Build history of the part. All positions in model axes, mm. Face numbers are marked on the shaded views. A direction names the side the tool comes from. Round coordinates to 2 decimals unless told otherwise and drop trailing zeros. Loops run counter-clockwise (first coordinate to the right, second up) from the corner with the lowest first, then second, coordinate; pieces in that order, holes last.
from build123d import *

# Parameters (mm, degrees)
SKETCH1_R           = 25
BOSS_EXTRUDE1_DEPTH = 50
SKETCH2_W           = 10
SKETCH2_H           = 10
BOSS_EXTRUDE2_DEPTH = 10
SKETCH3_R           = 2.5
BOSS_EXTRUDE3_DEPTH = 3
BOSS_EXTRUDE4_START = 3
SKETCH4_R           = 2.5
BOSS_EXTRUDE4_DEPTH = 3
CIRPATTERN1_COUNT   = 3
SKETCH5_R           = 7.5
SKETCH6_R           = 15
FILLET1_R           = 10
FILLET2_R           = 5


with BuildPart() as part:
    # Sketch1 → Boss-Extrude1 (new body)
    with BuildSketch(Plane.XY):
        Circle(SKETCH1_R)
    extrude(amount=BOSS_EXTRUDE1_DEPTH)

    # Sketch2 → Boss-Extrude2 (add)
    with BuildSketch(Plane(origin=(0, 0, 0), x_dir=(-1, 0, 0), z_dir=(0, 0, -1))):
        with Locations((29.494897428, 0)):
            Rectangle(SKETCH2_W, SKETCH2_H)
    boss_extrude2 = extrude(amount=-BOSS_EXTRUDE2_DEPTH)

    # Sketch3 → Boss-Extrude3 (add)
    with BuildSketch(Plane.XZ.offset(5)):
        with Locations((-29.494897428, 5)):
            Circle(SKETCH3_R)
    boss_extrude3 = extrude(amount=BOSS_EXTRUDE3_DEPTH)

    # Sketch4 → Boss-Extrude4 (add)
    with BuildSketch(Plane(origin=(0, 5, 0), x_dir=(1, 0, 0), z_dir=(0, 1, 0)).offset(BOSS_EXTRUDE4_START)):
        with Locations((-29.494897428, -5)):
            Circle(SKETCH4_R)
    boss_extrude4 = extrude(amount=-BOSS_EXTRUDE4_DEPTH)

    # CirPattern1: Boss-Extrude2, Boss-Extrude3, Boss-Extrude4 ×3 about axis
    cirpattern1_axis = Axis((0, 0, 0), (0, 0, 1))
    add([boss_extrude2.rotate(cirpattern1_axis, i * 360 / CIRPATTERN1_COUNT) for i in range(1, CIRPATTERN1_COUNT)])
    add([boss_extrude3.rotate(cirpattern1_axis, i * 360 / CIRPATTERN1_COUNT) for i in range(1, CIRPATTERN1_COUNT)])
    add([boss_extrude4.rotate(cirpattern1_axis, i * 360 / CIRPATTERN1_COUNT) for i in range(1, CIRPATTERN1_COUNT)])

    # Sketch5 → Cut-Loft1 section 0
    with BuildSketch(Plane.XY.offset(50)):
        Circle(SKETCH5_R)
    # Sketch6 → Cut-Loft1 section 1
    with BuildSketch(Plane(origin=(0, 0, 0), x_dir=(-1, 0, 0), z_dir=(0, 0, -1))):
        Circle(SKETCH6_R)
    loft(mode=Mode.SUBTRACT)

    # Fillet1
    fillet1_edges = [part.edges().sort_by_distance(p)[0] for p in [
        (-25, 0, 50),
    ]]
    fillet(fillet1_edges, radius=FILLET1_R)

    # Fillet2
    # the kernel refuses this fillet: 5 mm, written as the material it takes off along each edge
    with BuildSketch(Plane(origin=(0, 0, 0), x_dir=(0.22300738877667003, -0.9748167543446364, 0), z_dir=(-0.9748167543446364, -0.22300738877667003, 0))) as fillet2_piece_1_section:
        with BuildLine():
            CenterArc((25 - FILLET2_R, FILLET2_R), FILLET2_R, 270, 90)
            Line((25 - FILLET2_R, 0), (25, 0))
            Line((25, 0), (25, FILLET2_R))
        make_face()
    fillet2_piece_1 = revolve(axis=Axis((0, 0, 0), (0, 0, 1)), revolution_arc=77.11426693, mode=Mode.PRIVATE)
    fillet2_piece_1 = split(fillet2_piece_1, bisect_by=Plane(origin=(7.29782447, -22.640202767, 1.23109977), z_dir=(-0.8660254037844394, -0.49999999999999883, 0)), keep=Keep.TOP, mode=Mode.PRIVATE)
    add(fillet2_piece_1, mode=Mode.SUBTRACT)
    with BuildSketch(Plane(origin=(0, 0, 0), x_dir=(0.22300738877667003, -0.9748167543446364, 0), z_dir=(-0.9748167543446364, -0.22300738877667003, 0))) as fillet2_piece_2_section:
        with BuildLine():
            CenterArc((25 - FILLET2_R, FILLET2_R), FILLET2_R, 270, 90)
            Line((25 - FILLET2_R, 0), (25, 0))
            Line((25, 0), (25, FILLET2_R))
        make_face()
    fillet2_piece_2 = revolve(axis=Axis((0, 0, 0), (0, 0, 1)), revolution_arc=77.11426693, mode=Mode.PRIVATE)
    fillet2_piece_2 = split(fillet2_piece_2, bisect_by=Plane(origin=(13.725987665, -13.77410802, 1.168109868), z_dir=(0.8660254037844394, 0.4999999999999987, 0)), keep=Keep.TOP, mode=Mode.PRIVATE)
    add(fillet2_piece_2, mode=Mode.SUBTRACT)
    with BuildSketch(Plane(origin=(0, 0, 0), x_dir=(0.732831285228025, 0.68041039629847, 0), z_dir=(0.68041039629847, -0.732831285228025, 0))) as fillet2_piece_3_section:
        with BuildLine():
            CenterArc((25 - FILLET2_R, FILLET2_R), FILLET2_R, 270, 90)
            Line((25 - FILLET2_R, 0), (25, 0))
            Line((25, 0), (25, FILLET2_R))
        make_face()
    fillet2_piece_3 = revolve(axis=Axis((0, 0, 0), (0, 0, 1)), revolution_arc=154.248557626, mode=Mode.PRIVATE)
    fillet2_piece_3 = split(fillet2_piece_3, bisect_by=Plane(origin=(15.957681681, 17.639515442, 1.230959753), z_dir=(0.8660254037844378, -0.5000000000000014, 0)), keep=Keep.TOP, mode=Mode.PRIVATE)
    add(fillet2_piece_3, mode=Mode.SUBTRACT)
    with BuildSketch(Plane(origin=(0, 0, 0), x_dir=(0.732831285228025, 0.68041039629847, 0), z_dir=(0.68041039629847, -0.732831285228025, 0))) as fillet2_piece_4_section:
        with BuildLine():
            CenterArc((25 - FILLET2_R, FILLET2_R), FILLET2_R, 270, 90)
            Line((25 - FILLET2_R, 0), (25, 0))
            Line((25, 0), (25, FILLET2_R))
        make_face()
    fillet2_piece_4 = revolve(axis=Axis((0, 0, 0), (0, 0, 1)), revolution_arc=154.248557626, mode=Mode.PRIVATE)
    fillet2_piece_4 = split(fillet2_piece_4, bisect_by=Plane(origin=(1.564958422, 12.710587499, 1.419658234), z_dir=(-0.8660254037844378, 0.5000000000000017, 0)), keep=Keep.TOP, mode=Mode.PRIVATE)
    fillet2_piece_4 = split(fillet2_piece_4, bisect_by=Plane(origin=(-11.790170883, 5, 1.419658234), z_dir=(0, 1, 0)), keep=Keep.TOP, mode=Mode.PRIVATE)
    add(fillet2_piece_4, mode=Mode.SUBTRACT)
    with BuildSketch(Plane(origin=(0, 0, 0), x_dir=(0.732831285228025, 0.68041039629847, 0), z_dir=(0.68041039629847, -0.732831285228025, 0))) as fillet2_piece_5_section:
        with BuildLine():
            CenterArc((25 - FILLET2_R, FILLET2_R), FILLET2_R, 270, 90)
            Line((25 - FILLET2_R, 0), (25, 0))
            Line((25, 0), (25, FILLET2_R))
        make_face()
    fillet2_piece_5 = revolve(axis=Axis((0, 0, 0), (0, 0, 1)), revolution_arc=154.248557626, mode=Mode.PRIVATE)
    fillet2_piece_5 = split(fillet2_piece_5, bisect_by=Plane(origin=(-23.255109262, -5, 1.230959847), z_dir=(0, -1, 0)), keep=Keep.TOP, mode=Mode.PRIVATE)
    add(fillet2_piece_5, mode=Mode.SUBTRACT)
    with BuildSketch(Plane(origin=(0, 0, 0), x_dir=(-0.9556683308075251, 0.29444531154623416, 0), z_dir=(0.29444531154623416, 0.9556683308075251, 0))) as fillet2_piece_6_section:
        with BuildLine():
            CenterArc((25 - FILLET2_R, FILLET2_R), FILLET2_R, 270, 90)
            Line((25 - FILLET2_R, 0), (25, 0))
            Line((25, 0), (25, FILLET2_R))
        make_face()
    fillet2_piece_6 = revolve(axis=Axis((0, 0, 0), (0, 0, 1)), revolution_arc=154.248557626, mode=Mode.PRIVATE)
    fillet2_piece_6 = split(fillet2_piece_6, bisect_by=Plane(origin=(-23.255109324, 5, 1.230959753), z_dir=(0, 1, 0)), keep=Keep.TOP, mode=Mode.PRIVATE)
    add(fillet2_piece_6, mode=Mode.SUBTRACT)
    with BuildSketch(Plane(origin=(0, 0, 0), x_dir=(-0.9556683308075251, 0.29444531154623416, 0), z_dir=(0.29444531154623416, 0.9556683308075251, 0))) as fillet2_piece_7_section:
        with BuildLine():
            CenterArc((25 - FILLET2_R, FILLET2_R), FILLET2_R, 270, 90)
            Line((25 - FILLET2_R, 0), (25, 0))
            Line((25, 0), (25, FILLET2_R))
        make_face()
    fillet2_piece_7 = revolve(axis=Axis((0, 0, 0), (0, 0, 1)), revolution_arc=154.248557626, mode=Mode.PRIVATE)
    fillet2_piece_7 = split(fillet2_piece_7, bisect_by=Plane(origin=(1.564958422, -12.710587499, 1.419658234), z_dir=(-0.8660254037844394, -0.49999999999999883, 0)), keep=Keep.TOP, mode=Mode.PRIVATE)
    fillet2_piece_7 = split(fillet2_piece_7, bisect_by=Plane(origin=(-11.790170883, -5, 1.419658234), z_dir=(0, -1, 0)), keep=Keep.TOP, mode=Mode.PRIVATE)
    add(fillet2_piece_7, mode=Mode.SUBTRACT)
    with BuildSketch(Plane(origin=(0, 0, 0), x_dir=(-0.9556683308075251, 0.29444531154623416, 0), z_dir=(0.29444531154623416, 0.9556683308075251, 0))) as fillet2_piece_8_section:
        with BuildLine():
            CenterArc((25 - FILLET2_R, FILLET2_R), FILLET2_R, 270, 90)
            Line((25 - FILLET2_R, 0), (25, 0))
            Line((25, 0), (25, FILLET2_R))
        make_face()
    fillet2_piece_8 = revolve(axis=Axis((0, 0, 0), (0, 0, 1)), revolution_arc=154.248557626, mode=Mode.PRIVATE)
    fillet2_piece_8 = split(fillet2_piece_8, bisect_by=Plane(origin=(15.95768165, -17.639515389, 1.230959847), z_dir=(0.8660254037844394, 0.4999999999999987, 0)), keep=Keep.TOP, mode=Mode.PRIVATE)
    add(fillet2_piece_8, mode=Mode.SUBTRACT)
    with BuildSketch(Plane(origin=(0, 0, 0), x_dir=(1, 0, 0), z_dir=(0, -1, 0))) as fillet2_piece_9_section:
        with BuildLine():
            CenterArc((25 - FILLET2_R, FILLET2_R), FILLET2_R, 270, 90)
            Line((25 - FILLET2_R, 0), (25, 0))
            Line((25, 0), (25, FILLET2_R))
        make_face()
    fillet2_piece_9 = revolve(axis=Axis((0, 0, 0), (0, 0, 1)), revolution_arc=77.11426693, mode=Mode.PRIVATE)
    fillet2_piece_9 = split(fillet2_piece_9, bisect_by=Plane(origin=(13.725987546, 13.774107814, 1.168109699), z_dir=(0.8660254037844378, -0.5000000000000014, 0)), keep=Keep.TOP, mode=Mode.PRIVATE)
    add(fillet2_piece_9, mode=Mode.SUBTRACT)
    with BuildSketch(Plane(origin=(0, 0, 0), x_dir=(1, 0, 0), z_dir=(0, -1, 0))) as fillet2_piece_10_section:
        with BuildLine():
            CenterArc((25 - FILLET2_R, FILLET2_R), FILLET2_R, 270, 90)
            Line((25 - FILLET2_R, 0), (25, 0))
            Line((25, 0), (25, FILLET2_R))
        make_face()
    fillet2_piece_10 = revolve(axis=Axis((0, 0, 0), (0, 0, 1)), revolution_arc=77.11426693, mode=Mode.PRIVATE)
    fillet2_piece_10 = split(fillet2_piece_10, bisect_by=Plane(origin=(7.297824439, 22.640202713, 1.231099864), z_dir=(-0.8660254037844378, 0.5000000000000017, 0)), keep=Keep.TOP, mode=Mode.PRIVATE)
    add(fillet2_piece_10, mode=Mode.SUBTRACT)


solid = part.part
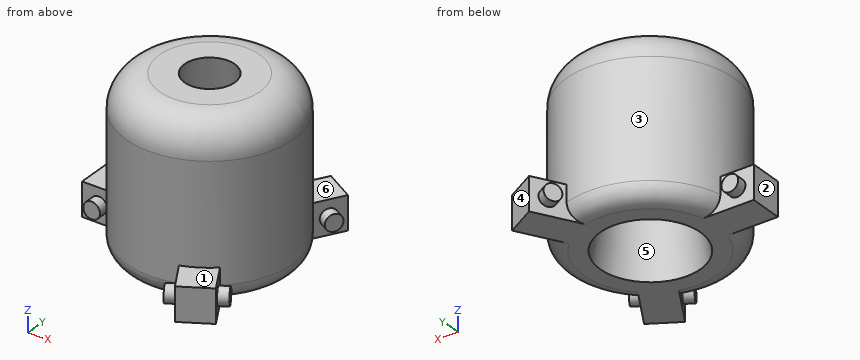
(1) Slice it at C-C on y = 6. Count the separate pieces of the cut face and the enclosed holes in it, plus the area to 3 significant figures.
Responses:
separate pieces: 3
enclosed holes: 0
area: 1,450 mm2
(2) Slice it at D-D on z = 26. List the corners of the cut face in (x, y), plus the area to 3 significant figures.
Responses:
outline: circle Ø50 at (0, 0); hole circle Ø22.2 at (0, 0)
area: 1,580 mm2
(3) Probe line 1 (Z direction, x = 15.5, y = 20.5); line 2 (X direction, y = 8, z = 12.5); line 3 (X direction, y = -6.5, z = 24). List the from-to ranges inside material, lowest first.
Responses:
line 1: z = 0 to 10
line 2: x = -23.69 to -10.41, 10.41 to 23.69
line 3: x = -24.14 to -9.37, 9.37 to 24.14
(4) Slice it at A-A on x = 0. List the corners of the cut face in (y, z).
Responses:
outline: (-25, 5) arc R5 ccw to (-20, 0) - (-15, 0) - (-7.5, 50) - (-15, 50) arc R10 ccw to (-25, 40) - close; (7.5, 50) - (15, 0) - (20, 0) arc R5 ccw to (25, 5) - (25, 40) arc R10 ccw to (15, 50) - close
(5) Slice it at B-B on z = 38. List the corners of the cut face in (x, y).
Responses:
outline: circle Ø50 at (0, 0); hole circle Ø18.6 at (0, 0)
(6) Pin check, flat tips, straight feed: P1, Ø3, axis at y = -8, z = 31, coming from the +X side; P2, Ø2, axis at x = 7, z = 28, coming from the -Y side; P3, Ø3, axis at x = -28, y = 2.5, coming from the +Z side; P4, Ø8, axis at x = -17.5, y = 24.5, coming from the +Z side. Stop position of each tip, or through.
Responses:
P1: stops at x = 24.14
P2: stops at y = -24.27
P3: stops at z = 10
P4: passes through
(7) Pull direction X, two halves, no side cores. Call the marked faces 4, 5 and 6: +X half, -X half, draft (parallel to the pull), parting line (faces both ways), or undercut.
Responses:
face 4: +X half
face 5: undercut
face 6: draft
(8) Which spindle directions (+Z, -Z, +X, -X, +Y, -Y) get a long thin tool onto all of the face, cutting with end or side? Do the marked faces 1, 2 and 3. Say none if no direction does.
Responses:
face 1: +Z, +X, -Y
face 2: +Z, -Z, -X, +Y, -Y
face 3: +Z
